Autodesk Inventor part; units mm, degrees
ref_plane "YZ Plane" through (0, 0, 0) normal (1, 0, 0) x (0, 1, 0)
ref_plane "XZ Plane" through (0, 0, 0) normal (0, 1, 0) x (-1, 0, 0)
ref_plane "XY Plane" through (0, 0, 0) normal (0, 0, 1) x (1, 0, 0)
sketch "Esboço1" plane through (0, 0, 0) normal (0, 0, 1) x (1, 0, 0)
  circle A0 centre (0, 0) radius 5.995 construction
  line L0 (13.9364, -15.0797) -> (-14.0636, -15.0797) construction
  line L1 (-14.0636, 14.3703) -> (13.9364, 14.3703)
  line L2 (13.9364, 14.3703) -> (13.9364, -15.0797)
  line L3 (13.9364, -15.0797) -> (-14.0636, -15.0797)
  line L4 (-14.0636, -15.0797) -> (-14.0636, 14.3703)
  circle A1 centre (0, 0) radius 6
  dimension "d0" = 12
extrude "Extrusão1" add sketch "Esboço1" along normal blind 20
sketch "Esboço2" plane through (-14.0636, 14.3703, 0) normal (0, 1, 0) x (1, 0, 0)
  line L0 (28, 0) -> (28, -20) construction
  line L1 (0, 0) -> (0, -20) construction
  line L2 (28, -10) -> (0, -10) construction
  line L3 (14, -10) -> (14, 0) construction
  line L4 (14, -10) -> (5.5, -10) construction
  line L5 (14, -10) -> (22.5, -10) construction
  dimension "d7" = 10
  dimension "d8" = 8.5
  dimension "d9" = 8.5
hole "Furo1" at (8.4364, 14.3703, 10) at (-8.5636, 14.3703, 10) direction (0, -1, 0) diameter 3.242 depth 8 tip angle 118
sketch "Esboço3" plane through (-14.0636, -15.0797, 0) normal (0, -1, 0) x (1, 0, 0)
  line L0 (28, 20) -> (0, 20)
  line L1 (14, 20) -> (14, 0) construction
  circle A0 centre (14, 10) radius 2
  point P0 (14.0636, 0)
  dimension "d17" = 20
  dimension "d18" = 4
hole "Furo2" at (-0.0636, -15.0797, 10) direction (0, 1, 0) diameter 3.242 depth 10 tip angle 118
properties part number "esbarro_carro" material "Alumínio 6061"
Could you check a few things on this model? Use its own coordinates, in mm. A direction names the side the tool comes from. Coordinates: 2 decimals unless noted, no trailing zeros. Order: outer loops, then holes, each group sorted by start corner. A loop starts at its lowest first (then second) coordinate and runs counter-clockwise, first axis right, second up. Notation, with made-up numbers: (-32.5, 24.5) - (6.5, 24.5) arc R19 ccw to (6.5, 49.5) - close; hole circle Ø2 at (-10.5, 16). An arc over 180 degrees is marked (long way). Answer in a Markdown table with one row per item. Add a question column.
(1) If we section it at B-B, the plane x = 3.5: Please give me the cut outline in (y, z), then the cut area to 3 significant figures.
(2) Will this pin go through, and if not, where does the flat tip stop? pin 1 (2.5 mm diameter, centred on x = -0.06, z = 10, fed in from -Y).
(3) I need wall thicknesses on L1, parallel to X at y = 8.75, z = 10; L2, parallel to Y at x = 0, z = 12.5; L3, parallel to X at y = -3.5, z = 12.75. Which ranges of each line are inside material? Lowest first, please.
(4) If we section it at C-C, the plane z = 17: Please give me the cut outline in (x, y).
(5) If we section it at D-D, the plane y = 10.5: Please give me the cut outline in (x, z).
(6) If we section it at A-A, the plane y = 0: Please give me the cut outline in (x, z).
(7) On a 3-axis mill with a long thin cutter (end or side, diameter ignored), from which of +Z, -Z, +X, -X, +Y, -Y can I reach the whole of each face in a straight line? I mean faces 4 (the face through (0, 14.37, 10)), 5 (the face through (-9.659, 10.314, 8.805)), 6 (the face through (-0.13, -10.35, 11.62)). Say none if no direction works.
(8) If we mould it in two halves opening along Z, with no side actions, what happens to faces 1 (the face through (-6.5, -0.1, 0)), 2 (the face through (-8.838, 5.565, 9.939)), 3 (the face through (-1.301, 5.857, 9.86))? For each: released by +Z, released by -Z, zero draft, split by the parting line, or undercut.
Results are:
| question | item | result |
|---|---|---|
| 1 | outline | (-15.08, 0) - (-4.87, 0) - (-4.87, 20) - (-15.08, 20) - close; (4.87, 0) - (14.37, 0) - (14.37, 20) - (4.87, 20) - close |
| 1 | area | 394 mm2 |
| 2 | pin 1 | stops at y = 5.86 |
| 3 | L1 | x = -14.06 to -10.18, -6.94 to 6.82, 10.06 to 13.94 |
| 3 | L2 | y = -15.08 to -6, 6 to 14.37 |
| 3 | L3 | x = -14.06 to -4.87, 4.87 to 13.94 |
| 4 | outline | (-14.06, -15.08) - (13.94, -15.08) - (13.94, 14.37) - (-14.06, 14.37) - close; hole circle Ø12 at (0, 0) |
| 5 | outline | (-14.06, 0) - (13.94, 0) - (13.94, 20) - (-14.06, 20) - close; hole circle Ø3.24 at (-8.56, 10); hole circle Ø3.24 at (8.44, 10) |
| 6 | outline | (-14.06, 0) - (-6, 0) - (-6, 20) - (-14.06, 20) - close; (6, 0) - (13.94, 0) - (13.94, 20) - (6, 20) - close |
| 7 | face 4 | +Z, -Z, +X, -X, +Y |
| 7 | face 5 | +Y |
| 7 | face 6 | -Y |
| 8 | face 1 | released by -Z |
| 8 | face 2 | undercut |
| 8 | face 3 | zero draft |
